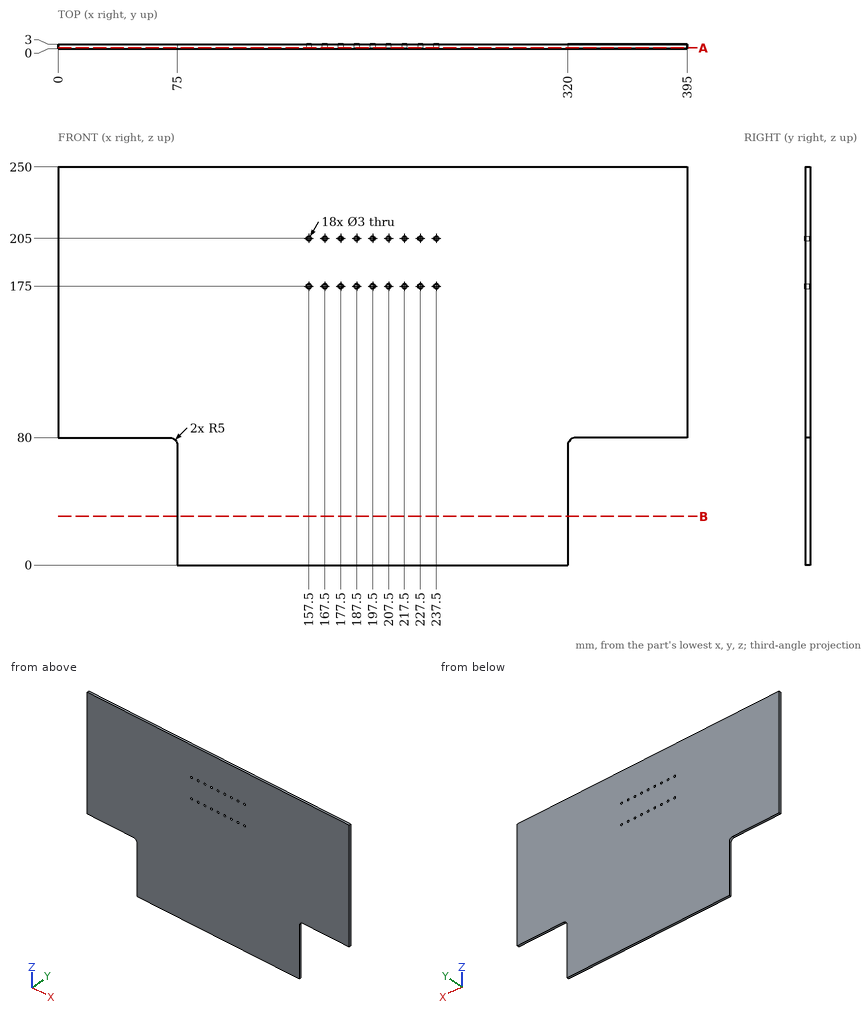
Part print with two shaded views. Sizes in mm from the minimum x, y, z corner. Coordinates: 2 decimals unless noted, no trailing zeros. Write each loop counter-clockwise with the first axis right and the second up, starting at its lowest first coordinate (ties: lowest second). Pieces come first, ordered by that corner, then holes. Notation, with made-up numbers: (-23, 1) - (-16, 1) arc R11 ccw to (-16, 9) - close; hole circle Ø11 at (51, 35.25). An arc over 180 degrees is marked (long way). Use a Markdown table: item, result. Add a question column.
Item 1: Drop flat-ended pins along their axis: pin 1 (5 mm diameter, centred on x = 163, z = 165.5, fed in from -Y); pin 2 (1.8 mm diameter, centred on x = 167.5, z = 205, fed in from +Y). Give the stop position or say it passes through.
Item 2: Band-saw the part on A-A, the plane y = 0.6. Give the number of separate pieces and of enclosed holes in the cut face, and give its area (3 significant figures).
Item 3: Band-saw the part on B-B, the plane z = 30.5. Write the cut outline in (x, y).
Item 4: Drill centre lines: line 1 along Z through (x, y) = (157.5, 0.9); line 2 along Z through (x, y) = (350.5, 1.75); line 3 along X through (y, z) = (2.6, 33). Where is each one in solid material? Low to high.
A:
| question | item | result |
|---|---|---|
| 1 | pin 1 | stops at y = 0 |
| 1 | pin 2 | passes through |
| 2 | separate pieces | 1 |
| 2 | enclosed holes | 18 |
| 2 | area | 86,600 mm² |
| 3 | outline | (75, 0) - (320, 0) - (320, 3) - (75, 3) - close |
| 4 | line 1 | z = 0 to 173.5, 176.5 to 203.5, 206.5 to 250 |
| 4 | line 2 | z = 80 to 250 |
| 4 | line 3 | x = 75 to 320 |
